Can you work these out from the model? Positions are in its coordinate system, mm. Face numbers are marked on the shaded views. A direction names the side the tool comes from. Give positions to 0.01 mm unless a question says otherwise; leave off trailing zeros. Write each loop counter-clockwise with the first axis right and the second up, starting at its lowest first coordinate (ties: lowest second). Pieces come first, ordered by that corner, then holes. Notation, with made-up numbers: (-9, -4) -> (22, -4) arc R13 ccw to (22, 9) -> close; hole circle Ø4 at (66.5, -19.75). An arc over 180 degrees is marked (long way). One line per item, written item: value.
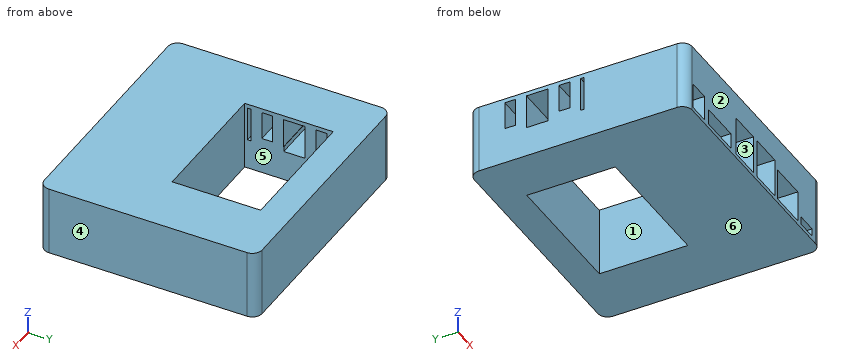
from build123d import *

# Parameters (mm, degrees)
SKETCH1_W           = 57.8
SKETCH1_H           = 38.4
BOSS_EXTRUDE1_DEPTH = 30
SKETCH2_W           = 8.89
SKETCH2_H           = 3.43
SKETCH2_W_2         = 14.05
SKETCH2_H_2         = 16.84
SKETCH2_W_3         = 17.696
SKETCH2_H_3         = 6.81
SKETCH2_W_4         = 9.3
SKETCH2_H_4         = 11
CUT_EXTRUDE1_DEPTH  = 23
SKETCH3_W           = 12.2
SKETCH3_H           = 4.7
CUT_EXTRUDE2_DEPTH  = 23


with BuildPart() as part:
    # Sketch1 → Boss-Extrude1 (new body)
    with BuildSketch(Plane.XY):
        with BuildLine():
            Line((84, 51.09), (-14.4, 51.09))
            ThreePointArc((-14.4, 51.09), (-17.440559159, 49.830559159), (-18.7, 46.79))
            Line((-18.7, 46.79), (-18.7, -39.11))
            ThreePointArc((-18.7, -39.11), (-17.440559159, -42.150559159), (-14.4, -43.41))
            Line((-14.4, -43.41), (84, -43.41))
            ThreePointArc((84, -43.41), (87.040559159, -42.150559159), (88.3, -39.11))
            Line((88.3, -39.11), (88.3, 46.79))
            ThreePointArc((88.3, 46.79), (87.040559159, 49.830559159), (84, 51.09))
        make_face()
        with Locations((32.8, 19.1)):
            Rectangle(SKETCH1_W, SKETCH1_H, mode=Mode.SUBTRACT)
    extrude(amount=-BOSS_EXTRUDE1_DEPTH)

    # Sketch2 → Cut-Extrude1 (cut)
    with BuildSketch(Plane.XZ.offset(43.41)):
        with Locations((76.775, -26.5048)):
            Rectangle(SKETCH2_W, SKETCH2_H)
        Polygon((66.12, -28.296), (68.12, -28.296), (69.827, -28.296), (69.827, -14.646007205), (68.12, -14.646007205), (66.12, -14.646007205), (57.38, -14.646007205), (55.38, -14.646007205), (53.673, -14.646007205), (53.673, -28.296), (55.38, -28.296), (57.38, -28.296), align=None)
        with Locations((44.4, -19.7998)):
            Rectangle(SKETCH2_W_2, SKETCH2_H_2)
        with Locations((27.4, -19.7998)):
            Rectangle(SKETCH2_W_2, SKETCH2_H_2)
        with Locations((7.56, -24.8148)):
            Rectangle(SKETCH2_W_3, SKETCH2_H_3)
        with Locations((-9.2, -22.796)):
            Rectangle(SKETCH2_W_4, SKETCH2_H_4)
    extrude(amount=-CUT_EXTRUDE1_DEPTH, mode=Mode.SUBTRACT)

    # Sketch3 → Cut-Extrude2 (cut)
    with BuildSketch(Plane.ZY.offset(18.7)):
        with Locations((-7.9, 33.2)):
            Rectangle(SKETCH3_W, SKETCH3_H)
        Polygon((-16.8, 26.15), (-1.8, 26.15), (-1.8, 16.75), (-14.6, 16.75), (-14.6, 16.875), (-16.8, 16.875), align=None)
        with Locations((-7.9, 9.7)):
            Rectangle(SKETCH3_W, SKETCH3_H)
        Polygon((-1.8, 1.1), (-16.8, 1.1), (-16.8, 2.7), (-1.8, 2.65), align=None)
    extrude(amount=-CUT_EXTRUDE2_DEPTH, mode=Mode.SUBTRACT)


solid = part.part
1) If we section it at B-B (x = 12.5): Write out the boundary of the cut face in (y, z), and give its area (3 significant figures).
Answer list:
outline: (-43.41, -30) -> (-0.1, -30) -> (-0.1, 0) -> (-43.41, 0) -> (-43.41, -21.41) -> (-20.41, -21.41) -> (-20.41, -28.22) -> (-43.41, -28.22) -> close; (38.3, -30) -> (51.09, -30) -> (51.09, 0) -> (38.3, 0) -> close
area: 1,530 mm^2
2) I need wall thicknesses on L1, parallel to X at y = -21, z = -23.75 (3 decimals); L2, parallel to Y at x = 7.5, z = -2.25; L3, parallel to X at y = 21.5, z = -23. Which ranges of each line are inside material? Lowest first, please.
Answer list:
L1: x = -18.7 to -13.85, -4.55 to -1.288, 16.408 to 20.375, 34.425 to 37.375, 51.425 to 53.673, 69.827 to 88.3
L2: y = -43.41 to -0.1, 38.3 to 51.09
L3: x = -18.7 to 3.9, 61.7 to 88.3
3) If we section it at D-D (z = -5.25): Write out the boundary of the cut face in (x, y).
Answer list:
outline: (-18.7, -39.11) arc R4.3 ccw to (-14.4, -43.41) -> (84, -43.41) arc R4.3 ccw to (88.3, -39.11) -> (88.3, 46.79) arc R4.3 ccw to (84, 51.09) -> (-14.4, 51.09) arc R4.3 ccw to (-18.7, 46.79) -> (-18.7, 35.55) -> (3.9, 35.55) -> (3.9, 38.3) -> (61.7, 38.3) -> (61.7, -0.1) -> (3.9, -0.1) -> (3.9, 1.1) -> (-18.7, 1.1) -> close; (-18.7, 2.66) -> (3.9, 2.66) -> (3.9, 7.35) -> (-18.7, 7.35) -> close; (-18.7, 12.05) -> (3.9, 12.05) -> (3.9, 16.75) -> (-18.7, 16.75) -> close; (-18.7, 26.15) -> (3.9, 26.15) -> (3.9, 30.85) -> (-18.7, 30.85) -> close
4) Will these pins go through, and if not, where does the flat tip stop? pin 1 (1.5 mm diameter, centred on x = 42.5, y = 2, fed in from -Z); pin 2 (7 mm diameter, centred on x = 61.5, z = -20, fed in from -Y).
Answer list:
pin 1: passes through
pin 2: stops at y = -20.41
5) We'd pull the mould along X, two halves only. Please class the marked faces 4, 5 and 6: released by +X, released by -X, zero draft, split by the parting line, or undercut.
Answer list:
face 4: released by +X
face 5: undercut
face 6: zero draft
6) For the marked faces 1, 2 and 3, which set-ups out of +Z, -Z, +X, -X, +Y, -Y let a thin tool reach every point of the face, with its end or its side?
Answer list:
face 1: +Z, -Z
face 2: +Z, -Z, +X, -X, -Y
face 3: -Y
7) If we section it at C-C (z = -19.25): Write out the boundary of the cut face in (x, y) (3 decimals).
Answer list:
outline: (-18.7, -39.11) arc R4.3 ccw to (-14.4, -43.41) -> (-13.85, -43.41) -> (-13.85, -20.41) -> (-4.55, -20.41) -> (-4.55, -43.41) -> (20.375, -43.41) -> (20.375, -20.41) -> (34.425, -20.41) -> (34.425, -43.41) -> (37.375, -43.41) -> (37.375, -20.41) -> (51.425, -20.41) -> (51.425, -43.41) -> (53.673, -43.41) -> (53.673, -20.41) -> (69.827, -20.41) -> (69.827, -43.41) -> (84, -43.41) arc R4.3 ccw to (88.3, -39.11) -> (88.3, 46.79) arc R4.3 ccw to (84, 51.09) -> (-14.4, 51.09) arc R4.3 ccw to (-18.7, 46.79) -> close; hole (3.9, -0.1) -> (61.7, -0.1) -> (61.7, 38.3) -> (3.9, 38.3) -> close
8) If we section it at A-A (y = 9): Write out the boundary of the cut face in (x, z), and give its area (3 significant figures).
Answer list:
outline: (-18.7, -30) -> (3.9, -30) -> (3.9, -14) -> (-18.7, -14) -> close; (-18.7, -1.8) -> (3.9, -1.8) -> (3.9, 0) -> (-18.7, 0) -> close; (61.7, -30) -> (88.3, -30) -> (88.3, 0) -> (61.7, 0) -> close
area: 1,200 mm^2
